Autodesk Fusion 360 part; units mm, degrees
sketch "Skizze1" plane through (0, 0, 0) normal (0, 0, 1) x (1, 0, 0)
  line L0 (74, -26) -> (-74, -26)
  line L1 (-74, -26) -> (-74, 26)
  line L2 (-74, 26) -> (74, 26)
  line L3 (74, 26) -> (74, -26)
  line L4 (74, -26) -> (-74, 26) construction
  line L5 (-74, -26) -> (74, 26) construction
  line L6 (-11.75, 61.7133) -> (-11.75, -53.3839) construction
  line L7 (-97.1763, 5.1) -> (112.5731, 5.1) construction
  line L8 (-53, 57.008) -> (-53, -45) construction
  line L9 (-95.9922, -11.9) -> (-35, -11.9) construction
  circle A0 centre (-53, -11.9) radius 4.5
  line L10 (-6.25, 0.35) -> (-17.25, 0.35)
  line L11 (-17.25, 0.35) -> (-17.25, 9.85)
  line L12 (-17.25, 9.85) -> (-6.25, 9.85)
  line L13 (-6.25, 9.85) -> (-6.25, 0.35)
  line L14 (-6.25, 0.35) -> (-17.25, 9.85) construction
  line L15 (-17.25, 0.35) -> (-6.25, 9.85) construction
  point P0 (-53, -11.9)
  point P1 (-11.75, 5.1)
  dimension "d1" = 148
  dimension "d2" = 52
  dimension "d3" = 62.25
  dimension "d4" = 20.9
  dimension "d6" = 21
  dimension "d8" = 37.9
  dimension "d9" = 9
  dimension "d12" = 11
  dimension "d13" = 9.5
extrude "Extrusion1" add sketch "Skizze1" along normal blind 2
Can you work these out from the model? Positions are in its coordinate system, mm. Give positions to 0.01 mm unless a question says otherwise; leave off trailing zeros. Write each loop counter-clockwise with the first axis right and the second up, starting at its lowest first coordinate (ties: lowest second). Pieces come first, ordered by that corner, then holes. Notation, with made-up numbers: (57.25, 80.5) - (74.25, 80.5) arc R24 cw to (74.25, 118.5) - close; hole circle Ø5 at (16.5, -4.5). An arc over 180 degrees is marked (long way). Write item = value, one per line. Start each with the question number.
1. Imagine slicing it at B-B (x = -53). Please give me the cut outline in (y, z).
2. For pin 1 (3 mm diameter, centred on x = -8.5, y = 5.5, fed in from -Z), with a flat end and sliding along its axis, tell me the tip position at first contact or that it passes through.
3. Please list where these lines run through material, in increasing order: line 1 (Y direction, x = -53, z = 1.2); line 2 (Y direction, x = -16.5, z = 0.4).
4. Imagine slicing it at C-C (z = 1.35). Please give me the cut outline in (x, y).
5. Imagine slicing it at A-A (y = 6.5). Please give me the cut outline in (x, z), and give its area (3 significant figures).
6. Thinking about a two-plate mould opening in Y: for faces 1 (the face through (-50.92, -7.91, 0.99)), 2 (the face through (-1, 0, 0)), which applies, released by +Y, released by -Y, zero draft, split by the parting line, or undercut?
Worked answers:
q1.outline = (-26, 0) - (-16.4, 0) - (-16.4, 2) - (-26, 2) - close; (-7.4, 0) - (26, 0) - (26, 2) - (-7.4, 2) - close
q2.pin_1 = through
q3.line_1 = -26 to -16.4, -7.4 to 26
q3.line_2 = -26 to 0.35, 9.85 to 26
q4.outline = (-74, -26) - (74, -26) - (74, 26) - (-74, 26) - close; hole circle Ø9 at (-53, -11.9); hole (-17.25, 0.35) - (-6.25, 0.35) - (-6.25, 9.85) - (-17.25, 9.85) - close
q5.outline = (-74, 0) - (-17.25, 0) - (-17.25, 2) - (-74, 2) - close; (-6.25, 0) - (74, 0) - (74, 2) - (-6.25, 2) - close
q5.area = 274 mm2
q6.face_1 = undercut
q6.face_2 = zero draft
